from build123d import *

# Parameters (mm, degrees)
F1_DEPTH       = 26
F3_D           = 6.4
F5_D           = 6
F5_DEPTH       = 46
F5_START       = 5
F5_CBORE_D     = 11
F5_CBORE_DEPTH = 6
F5_TIP         = 1.8025818571


with BuildPart() as f1:
    # F0 (on Right) → F1 (new body)
    with BuildSketch(Plane.YZ):
        with BuildLine():
            Line((-33.5, 6.5), (-27, 0))
            Line((-27, 0), (27, 0))
            Line((27, 0), (33.5, 6.5))
            Line((33.5, 6.5), (33.5, 25))
            Line((33.5, 25), (21.4767315949, 25))
            ThreePointArc((21.4767315949, 25), (-21.5, 26), (21.4767315949, 27))
            Line((21.4767315949, 27), (33.5, 27))
            Line((33.5, 27), (33.5, 45))
            Line((33.5, 45), (47.5, 45))
            Line((47.5, 45), (47.5, 63))
            Line((47.5, 63), (-47.5, 63))
            Line((-47.5, 63), (-47.5, 45))
            Line((-47.5, 45), (-33.5, 45))
            Line((-33.5, 45), (-33.5, 6.5))
        make_face()
    extrude(amount=F1_DEPTH)

    # F3 (through all)
    with Locations(Plane(origin=(0, 0, 45), x_dir=(1, 0, 0), z_dir=(0, 0, -1))):
        with Locations((6, 40), (20, 40), (20, -40), (6, -40)):
            Hole(F3_D / 2)

    # F5
    # its depths count from where the whole tool has entered the part; down to there all is cleared
    with Locations(Plane(origin=(0, 0, 0), x_dir=(1, 0, 0), z_dir=(0, 0, -1)).offset(-F5_START)):
        with Locations((13, -26.5)):
            CounterBoreHole(F5_D / 2, F5_CBORE_D / 2, F5_CBORE_DEPTH, depth=F5_DEPTH)
            with Locations((0, 0, -(F5_DEPTH + F5_TIP / 2))):  # 118° drill point
                Cone(0, F5_D / 2, F5_TIP, mode=Mode.SUBTRACT)


solid = f1.part
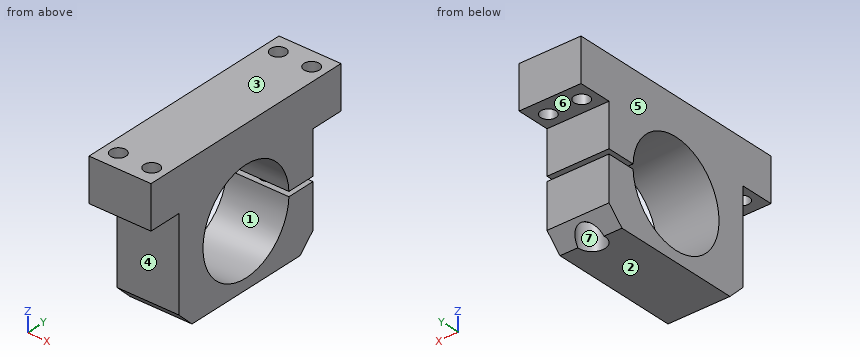
Could you check a few things on this model? Use its own coordinates, in mm. Face numbers are marked on the shaded views. A direction names the side the tool comes from. Round coordinates to 2 decimals unless told otherwise and drop trailing zeros. Order: outer loops, then holes, each group sorted by start corner. A loop starts at its lowest first (then second) coordinate and runs counter-clockwise, first axis right, second up. Notation, with made-up numbers: M 38.5,-4.5 L 79.5,-4.5 A36 ccw 79.5,34.5 Z; hole C 88.25,-17.5 d10. An arc over 180 degrees is marked long. One line per item, written item: value.
(1) Imagine slicing it at C-C (x = 20). Write out the boundary of the cut face in (y, z).
Ans:
outline: M -47.5,45 L -43.2,45 L -43.2,63 L -47.5,63 Z; M -36.8,45 L -33.5,45 L -33.5,6.5 L -27,0 L 27,0 L 33.5,6.5 L 33.5,25 L 21.48,25 A21.5 cw long 21.48,27 L 33.5,27 L 33.5,45 L 36.8,45 L 36.8,63 L -36.8,63 Z; M 43.2,45 L 47.5,45 L 47.5,63 L 43.2,63 Z
(2) If we mould it in two halves opening along Z, with no side actions, what happens to the marked faces 1, 2, 3 and 4? For each: released by +Z, released by -Z, zero draft, split by the parting line, or undercut.
Ans:
face 1: undercut
face 2: released by -Z
face 3: released by +Z
face 4: zero draft
(3) I need wall thicknesses on line 1 along Y through (x, z) = (20, 51.5); line 2 along X through (y, z) = (40, 56); line 3 along Z through (x, y) = (10, 0). Which ranges of each line are inside material? Lowest first, please. Write a range as from..to.
Ans:
line 1: y = -47.5..-43.2, -36.8..36.8, 43.2..47.5
line 2: x = 0..2.8, 9.2..16.8, 23.2..26
line 3: z = 0..4.5, 47.5..63
(4) I'm going to push flat-ended pins straight in: P1, Ø3.5, axis at x = 11.5, y = 26.5, coming from the -Z side; P2, Ø7.5, axis at x = 6, y = -40, coming from the -Z side; P3, Ø9, axis at x = 13, z = 34, coming from the +Y side. Where does each tip first touch, or does it pass through?
Ans:
P1: stops at z = 11
P2: stops at z = 45
P3: stops at y = 33.5
(5) Imagine slicing it at B-B (y = 0). Write out the boundary of the cut face in (x, z), and give its area (3 significant figures).
Ans:
outline: M 0,0 L 26,0 L 26,4.5 L 0,4.5 Z; M 0,47.5 L 26,47.5 L 26,63 L 0,63 Z
area: 520 mm^2
(6) Which directions (+Z, -Z, +X, -X, +Y, -Y) give clear straight access to the entire face, cutting with the end or side of a thin tool? Please do the marked faces 5, 6 and 7.
Ans:
face 5: +Z, -Z, -X, +Y, -Y
face 6: -Z, +X, -X, +Y
face 7: -Z
(7) Imagine slicing it at A-A (z = 10). Write out the boundary of the cut face in (x, y).
Ans:
outline: M 0,-33.5 L 26,-33.5 L 26,-14.36 L 0,-14.36 Z; M 0,14.36 L 26,14.36 L 26,33.5 L 0,33.5 Z; hole C 13,26.5 d11
(8) Imagine slicing it at D-D (y = 40). Write out the boundary of the cut face in (x, z).
Ans:
outline: M 0,45 L 2.8,45 L 2.8,63 L 0,63 Z; M 9.2,45 L 16.8,45 L 16.8,63 L 9.2,63 Z; M 23.2,45 L 26,45 L 26,63 L 23.2,63 Z
